The model under review builds one solid part; all positions refer to its coordinate system, in mm. Face numbers are marked on the shaded views. A direction names the side the tool comes from. Round coordinates to 2 decimals unless told otherwise and drop trailing zeros. Loops run counter-clockwise (first coordinate to the right, second up) from the corner with the lowest first, then second, coordinate; pieces in that order, holes last. Notation, with made-up numbers: M 43.5,-7 L 63.5,-7 A9 ccw 63.5,9 Z; hole C 2.5,75 d5. An arc over 180 degrees is marked long. Return JSON: item names as keys, results as strings. Group by question number.
Q1. For the marked faces 1 and 2, list the 3-axis set-ups (+Z, -Z, +X, -X, +Y, -Y) from which the entire face can be reached by the end or side of a thin tool; tool diameter is ignored.
Q2. Draft analysis for pull direction Y (two halves, no side actions). For the marked faces 3, 4 and 5, state which applies: pulls with the +Y half, pulls with the -Y half, needs draft (parallel to the pull), parting line crosses it, or undercut.
Q3. Clearance check with flat-ended pins moving along their axes: pin 1 Ø12 at (x, y) = (13.5, 40) entering from +Z; pin 2 Ø1.2 at (y, z) = (-3.5, 12.5) entering from +X; pin 3 Ø2.5 at (y, z) = (-4, 9.5) entering from +X. State where each tip first meets the part, or that it passes through.
Q4. Consider section B-B (x = 47.5). State the section outline as (y, z) points, and give its area (4 significant figures).
Q5. To check wall thickness, follow line 1 along X through (y, z) = (69, 11.5); line 2 along Y through (x, z) = (57, 20.25); line 3 along Z through (x, y) = (7.5, 16.5). State the ranges of each line that lie inside material, in increasing order.
Q6. Consider section A-A (z = 23). State the section outline as (x, y) points, and give its area (3 significant figures).
Q7. Consider section C-C (z = 9.5). State the section outline as (x, y) points.
Q8. Consider section D-D (y = 29.5). State the section outline as (x, z) points, and give its area (4 significant figures).
from build123d import *

# Parameters (mm, degrees)
F0_W     = 58
F0_H     = 82
F1_DEPTH = 19
F2_W     = 67.999994
F2_H     = 91.999994
F3_DEPTH = 25
F4_R     = 5
F5_T     = -2.5
F6_W     = 10
F6_H     = 8
F6_R     = 6
F7_DEPTH = 25


with BuildPart() as f1:
    # F0 (on Top) → F1 (new body)
    with BuildSketch(Plane.XY):
        with Locations((29, 41)):
            Rectangle(F0_W, F0_H)
    extrude(amount=F1_DEPTH)


with BuildPart() as f3:
    # F2 (on Top) → F3 (new body)
    with BuildSketch(Plane.XY):
        with Locations((29, 41)):
            Rectangle(F2_W, F2_H)
    extrude(amount=F3_DEPTH)

    # F4
    f4_edges = [f3.edges().sort_by_distance(p)[0] for p in [
        (-4.999997, -4.999997, 12.5),
        (62.999997, -4.999997, 12.5),
        (-4.999997, 86.999997, 12.5),
        (62.999997, 86.999997, 12.5),
    ]]
    fillet(f4_edges, radius=F4_R)

    # F5
    f5_openings = [f3.faces().sort_by_distance(p)[0] for p in [
        (29, 41, 25),
    ]]
    offset(amount=F5_T, openings=f5_openings)


with BuildPart() as f7_tool:
    # F6 (on face) → F7 (new body)
    with BuildSketch(Plane.XZ.offset(4.999997)):
        with Locations((21.000003, 11.4)):
            Rectangle(F6_W, F6_H)
        with Locations((33.000003, 11.4)):
            Circle(F6_R)
        with Locations((45.000003, 11.4)):
            Rectangle(F6_W, F6_H)
    extrude(amount=-F7_DEPTH)


with BuildPart() as f1_1:
    add(f1.part)

    # F7: cut by f7_tool
    add(f7_tool.part, mode=Mode.SUBTRACT)


with BuildPart() as f3_1:
    add(f3.part)

    # F7: cut by f7_tool
    add(f7_tool.part, mode=Mode.SUBTRACT)


solid = f3_1.part
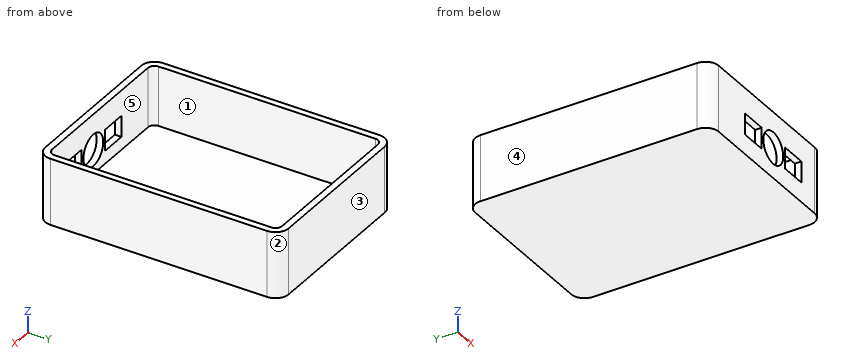
Values:
{
 "1": {"face 1": "+Z", "face 2": "+Z, -Z, +X, +Y"},
 "2": {"face 3": "pulls with the +Y half", "face 4": "needs draft", "face 5": "undercut"},
 "3": {"pin 1": "stops at z = 2.5", "pin 2": "stops at x = 62.07", "pin 3": "stops at x = 62.18"},
 "4": {"outline": "M -5,0 L 87,0 L 87,25 L 84.5,25 L 84.5,2.5 L -2.5,2.5 L -2.5,7.4 L -5,7.4 Z; M -5,15.4 L -2.5,15.4 L -2.5,25 L -5,25 Z", "area": "322.5 mm2"},
 "5": {"line 1": "x = -5 to -2.5, 60.5 to 63", "line 2": "y = -5 to -2.5, 84.5 to 87", "line 3": "z = 0 to 2.5"},
 "6": {"outline": "M -5,0 A5 ccw 0,-5 L 58,-5 A5 ccw 63,0 L 63,82 A5 ccw 58,87 L 0,87 A5 ccw -5,82 Z; hole M -2.5,0 A2.5 ccw 0,-2.5 L 58,-2.5 A2.5 ccw 60.5,0 L 60.5,82 A2.5 ccw 58,84.5 L 0,84.5 A2.5 ccw -2.5,82 Z", "area": "759 mm2"},
 "7": {"outline": "M -5,0 A5 ccw 0,-5 L 16,-5 L 16,-2.5 L 0,-2.5 A2.5 cw -2.5,0 L -2.5,82 A2.5 cw 0,84.5 L 58,84.5 A2.5 cw 60.5,82 L 60.5,0 A2.5 cw 58,-2.5 L 50,-2.5 L 50,-5 L 58,-5 A5 ccw 63,0 L 63,82 A5 ccw 58,87 L 0,87 A5 ccw -5,82 Z; M 26,-5 L 27.31,-5 L 27.31,-2.5 L 26,-2.5 Z; M 38.69,-5 L 40,-5 L 40,-2.5 L 38.69,-2.5 Z"},
 "8": {"outline": "M -5,0 L 63,0 L 63,25 L 60.5,25 L 60.5,2.5 L -2.5,2.5 L -2.5,25 L -5,25 Z", "area": "282.5 mm2"}
}
